Input: part model. Units: mm. Frame: model coordinates. A direction names the side the tool comes from. Give positions to 0.01 mm unless a question says otherwise; leave off trailing zeros. Order: outer loops, then holes, each group sorted by start corner. A loop starts at its lowest first (then second) coordinate and runs counter-clockwise, first axis right, second up. Notation, with made-up numbers: (-16, 54.25) - (-9, 54.25) arc R10 ccw to (-9, 73.25) - close; hole circle Ø2 at (-10.75, 36.25). An arc over 180 degrees is marked (long way). Answer in a Markdown table with one row per item. Add a question column.
1. Contact query for flat-ended pins moving along their axis: pin 1 (8 mm diameter, centred on x = 31, z = 31.5, fed in from -Y); pin 2 (1 mm diameter, centred on x = 1.5, z = 23, fed in from +Y); pin 3 (1 mm diameter, centred on x = 22, z = 5, fed in from +Y); pin 4 (4 mm diameter, centred on x = 24, y = 32, fed in from -Z) (3 decimals). Output: stop coordinate, or through.
2. Section query D-D on x = -24. Count the separate pieces of the cut face and the enclosed holes in it, and give its area (3 significant figures).
3. Access query for faces 5 (the face through (15.7, 15, 3.5)), 6 (the face through (-37.785, 0.234, 32.233)), 7 (the face through (-36, -12.15, 34)). Directions: +Z, -Z, +X, -X, +Y, -Y. A direction counts if a zero-diameter tool reaches every point of the face in a straight line with its end or side. Return the directions, or none.
4. Section query B-B on z = 6.5. Return loops of the section in (x, y), and give its area (4 significant figures).
5. Section query A-A on x = 24. Return loops of the section in (y, z), and give its area (3 significant figures).
6. Ray query, line 1 (Y direction, x = -36, z = 32.15); line 2 (X direction, y = -15, z = 32); line 3 (Y direction, x = 4, z = 9). Return the intervals inside material, ascending. Write a range as [from, to].
7. Mould query, pull axis Z, two halves, no side actions, for faces 1 (the face through (-23.72, 34.134, 1.25)), 2 (the face through (27.7, 15, 3.5)), 3 (the face through (-22, -34, 2.536)), 4 (the face through (-38, -15, 32.8)). Classes: released by +Z, released by -Z, zero draft, split by the parting line, or undercut.
8. Section query C-C on y = 11. Return loops of the section in (x, z), and give its area (4 significant figures).
```python
from build123d import *

# Parameters (mm, degrees)
ESQUISSE3_W                                        = 80
ESQUISSE3_H                                        = 52
BOSS_EXTRU_1_DEPTH                                 = 5
ESQUISSE4_R                                        = 6.4
ENL_V_MAT_EXTRU_1_DEPTH                            = 10
BOSS_EXTRU_2_DEPTH                                 = 33
CHAMBRAGE_POUR_VIS_T_TE_RONDE_BOMB_E_M_D           = 3.1
CHAMBRAGE_POUR_VIS_T_TE_RONDE_BOMB_E_M_CBORE_D     = 6
CHAMBRAGE_POUR_VIS_T_TE_RONDE_BOMB_E_M_CBORE_DEPTH = 3.5
R_P_TITION_LIN_AIRE1_COUNT                         = 2
R_P_TITION_LIN_AIRE1_PITCH                         = 12
R_P_TITION_LIN_AIRE1_COUNT_DIR2                    = 2
R_P_TITION_LIN_AIRE1_PITCH_DIR2                    = 24
ENL_V_MAT_EXTRU_2_REACH                            = 94.304
ESQUISSE11_W                                       = 2.5
ESQUISSE11_H                                       = 5.7
R_P_TITION_LIN_AIRE2_COUNT                         = 3
R_P_TITION_LIN_AIRE2_PITCH                         = 15
R_P_TITION_LIN_AIRE3_COUNT                         = 3
R_P_TITION_LIN_AIRE3_PITCH                         = 15
BOSS_EXTRU_3_DEPTH                                 = 5
CHAMBRAGE_POUR_VIS_T_TE_RONDE_BOMB_E_D             = 4.3053
CHAMBRAGE_POUR_VIS_T_TE_RONDE_BOMB_E_CBORE_D       = 7.54126
CHAMBRAGE_POUR_VIS_T_TE_RONDE_BOMB_E_CBORE_DEPTH   = 2.4638
ESQUISSE19_W                                       = 2.951567909
ESQUISSE19_H                                       = 7.383496099
ENL_V_MAT_EXTRU_3_DEPTH                            = 1


with BuildPart() as part:
    # Esquisse3 → Boss.-Extru.1 (new body)
    with BuildSketch(Plane.XY):
        Rectangle(ESQUISSE3_W, ESQUISSE3_H)
    extrude(amount=BOSS_EXTRU_1_DEPTH)

    # Esquisse4 → Enlèv. mat.-Extru.1 (cut)
    with BuildSketch(Plane.XY.offset(5)):
        with Locations((-22, -12)):
            Circle(ESQUISSE4_R)
    extrude(amount=-ENL_V_MAT_EXTRU_1_DEPTH, mode=Mode.SUBTRACT)

    # Esquisse5 → Boss.-Extru.2 (add)
    with BuildSketch(Plane.XY.offset(5)):
        Polygon((-40, -26), (40, -26), (40, -23.5), (-32.5, -23.5), (-32.5, 23.5), (40, 23.5), (40, 26), (-40, 26), align=None)
    extrude(amount=BOSS_EXTRU_2_DEPTH)

    # Chambrage pour vis à tête ronde bombée M2.51 (through all)
    with Locations(Plane(origin=(0, 0, 0), x_dir=(-1, 0, 0), z_dir=(0, 0, -1))):
        with Locations((-17, 16.25)):
            chambrage_pour_vis_t_te_ronde_bomb_e_m = CounterBoreHole(CHAMBRAGE_POUR_VIS_T_TE_RONDE_BOMB_E_M_D / 2, CHAMBRAGE_POUR_VIS_T_TE_RONDE_BOMB_E_M_CBORE_D / 2, CHAMBRAGE_POUR_VIS_T_TE_RONDE_BOMB_E_M_CBORE_DEPTH)

    # Répétition linéaire1: Chambrage pour vis à tête ronde bombée #61 M 2 × 2
    with Locations(*[(i * R_P_TITION_LIN_AIRE1_PITCH, -j * R_P_TITION_LIN_AIRE1_PITCH_DIR2, 0) for i in range(R_P_TITION_LIN_AIRE1_COUNT) for j in range(R_P_TITION_LIN_AIRE1_COUNT_DIR2) if (i, j) != (0, 0)]):
        add(chambrage_pour_vis_t_te_ronde_bomb_e_m, mode=Mode.SUBTRACT)

    # Esquisse11 → Enlèv. mat.-Extru.2 (cut, up to next)
    with BuildSketch(Plane.ZY.offset(40), mode=Mode.PRIVATE) as enl_v_mat_extru_2_sk1:
        with Locations((34.05, 15)):
            Rectangle(ESQUISSE11_W, ESQUISSE11_H)
    enl_v_mat_extru_2_tool1 = extrude(enl_v_mat_extru_2_sk1.sketch, amount=-ENL_V_MAT_EXTRU_2_REACH, mode=Mode.PRIVATE) & part.part
    enl_v_mat_extru_2 = enl_v_mat_extru_2_tool1.solids().sort_by_distance((-40, 15, 34.05))[0]
    add(enl_v_mat_extru_2, mode=Mode.SUBTRACT)

    # Répétition linéaire2: Enlèv. mat.-Extru.2 ×3
    with Locations(*[(0, -i * R_P_TITION_LIN_AIRE2_PITCH, 0) for i in range(1, R_P_TITION_LIN_AIRE2_COUNT)]):
        add(enl_v_mat_extru_2, mode=Mode.SUBTRACT)

    # Esquisse15 → Dégagement M31 (revolve, cut)
    with BuildSketch(Plane(origin=(-36, 15, 38), x_dir=(0, -1, 0), z_dir=(1, 0, 0))):
        Polygon((0, 0), (0, 7.431549114), (1.8, 6.35), (1.8, 0), align=None)
    d_gagement_m31 = revolve(axis=Axis((-36, 15, 44.35), (0, 0, -1)), mode=Mode.SUBTRACT)

    # Répétition linéaire3: Dégagement M31 ×3
    with Locations(*[(0, -i * R_P_TITION_LIN_AIRE3_PITCH, 0) for i in range(1, R_P_TITION_LIN_AIRE3_COUNT)]):
        add(d_gagement_m31, mode=Mode.SUBTRACT)

    # Esquisse16 → Boss.-Extru.3 (add)
    with BuildSketch(Plane(origin=(0, 0, 0), x_dir=(-1, 0, 0), z_dir=(0, 0, -1))):
        with BuildLine():
            Line((-35, 26), (-13, 26))
            ThreePointArc((-13, 26), (-17.242640687, 27.757359313), (-19, 32))
            ThreePointArc((-19, 32), (-24, 37), (-29, 32))
            ThreePointArc((-29, 32), (-30.757359313, 27.757359313), (-35, 26))
        make_face()
        with BuildLine():
            Line((13, 26), (35, 26))
            ThreePointArc((35, 26), (30.757359313, 27.757359313), (29, 32))
            ThreePointArc((29, 32), (24, 37), (19, 32))
            ThreePointArc((19, 32), (17.242640687, 27.757359313), (13, 26))
        make_face()
        with BuildLine():
            Line((-35, -26), (-13, -26))
            ThreePointArc((-13, -26), (-17.242640687, -27.757359313), (-19, -32))
            ThreePointArc((-19, -32), (-24, -37), (-29, -32))
            ThreePointArc((-29, -32), (-30.757359313, -27.757359313), (-35, -26))
        make_face()
        with BuildLine():
            Line((13, -26), (35, -26))
            ThreePointArc((35, -26), (30.757359313, -27.757359313), (29, -32))
            ThreePointArc((29, -32), (24, -37), (19, -32))
            ThreePointArc((19, -32), (17.242640687, -27.757359313), (13, -26))
        make_face()
    extrude(amount=-BOSS_EXTRU_3_DEPTH)

    # Chambrage pour vis à tête ronde bombée #61 (through all)
    with Locations(Plane.XY.offset(5)):
        with Locations((-24, 32), (24, 32), (24, -32), (-24, -32)):
            CounterBoreHole(CHAMBRAGE_POUR_VIS_T_TE_RONDE_BOMB_E_D / 2, CHAMBRAGE_POUR_VIS_T_TE_RONDE_BOMB_E_CBORE_D / 2, CHAMBRAGE_POUR_VIS_T_TE_RONDE_BOMB_E_CBORE_DEPTH)

    # Esquisse19 → Enlèv. mat.-Extru.3 (cut)
    with BuildSketch(Plane(origin=(-32.5, 0, 0), x_dir=(0, 0, -1), z_dir=(1, 0, 0))):
        with Locations((-26.438573375, -11.379122074)):
            Rectangle(ESQUISSE19_W, ESQUISSE19_H)
    extrude(amount=-ENL_V_MAT_EXTRU_3_DEPTH, mode=Mode.SUBTRACT)


solid = part.part
```
Answer:
| question | item | result |
|---|---|---|
| 1 | pin 1 | stops at y = -26 |
| 1 | pin 2 | stops at y = 26 |
| 1 | pin 3 | stops at y = 36.77 |
| 1 | pin 4 | passes through |
| 2 | separate pieces | 4 |
| 2 | enclosed holes | 0 |
| 2 | area | 415 mm² |
| 3 | face 5 | -Z |
| 3 | face 6 | +Z |
| 3 | face 7 | +X, -X |
| 4 | outline | (-40, -26) - (40, -26) - (40, -23.5) - (-32.5, -23.5) - (-32.5, 23.5) - (40, 23.5) - (40, 26) - (-40, 26) - close |
| 4 | area | 752.5 mm² |
| 5 | outline | (-37, 0) - (-34.15, 0) - (-34.15, 2.54) - (-35.77, 2.54) - (-35.77, 5) - (-37, 5) - close; (-29.85, 0) - (29.85, 0) - (29.85, 2.54) - (28.23, 2.54) - (28.23, 5) - (26, 5) - (26, 38) - (23.5, 38) - (23.5, 5) - (-23.5, 5) - (-23.5, 38) - (-26, 38) - (-26, 5) - (-28.23, 5) - (-28.23, 2.54) - (-29.85, 2.54) - close; (34.15, 0) - (37, 0) - (37, 5) - (35.77, 5) - (35.77, 2.54) - (34.15, 2.54) - close |
| 5 | area | 476 mm² |
| 6 | line 1 | y = [-26, -16.8], [-13.2, -1.8], [1.8, 13.2], [16.8, 26] |
| 6 | line 2 | x = [-40, -37.8], [-34.2, -32.5] |
| 6 | line 3 | y = [-26, -23.5], [23.5, 26] |
| 7 | face 1 | zero draft |
| 7 | face 2 | released by -Z |
| 7 | face 3 | released by +Z |
| 7 | face 4 | undercut |
| 8 | outline | (-40, 0) - (40, 0) - (40, 5) - (-32.5, 5) - (-32.5, 38) - (-40, 38) - close |
| 8 | area | 647.5 mm² |
